Source: CAD feature listing. Evaluate the final solid. Frame: model axes, mm. Give positions to 0.01 mm unless a question says otherwise; leave off trailing zeros. Order: outer loops, then holes, each group sorted by start corner. A loop starts at its lowest first (then second) coordinate and runs counter-clockwise, first axis right, second up.
1) Section A-A, the plane x = 0. Return loops of the section in (y, z).
2) Section B-B, the plane z = 5.5. Return loops of the section in (x, y), plus the area to 3 significant figures.
3) Draft query along X for faces 1 (the face through (-2, 3.5, -2)), 2 (the face through (1.07, 1.73, -8.13)), 3 (the face through (-3, 2, 3)). Return one class per face: released by +X, released by -X, zero draft, split by the parting line, or undercut.
4) Material intervals for line 1 (Z direction, x = 0, y = 1.95); line 2 (X direction, y = 1.4, z = 6); line 3 (X direction, y = 2.25, z = 1.5), sorted ascending.
5) First-contact query: P1, Ø2, axis at x = 3.5, y = 1, coming from the +Z side; P2, Ø1, axis at x = -3.5, y = 2.5, coming from the +Z side. Flat tips, straight axial feed; report the tip coordinate or a pass-through.
6) Section D-D, the plane y = 2.35. Give the number of separate pieces and of enclosed holes in the cut face, plus the area to 3 significant figures.
7) Section C-C, the plane z = -3.75. Return loops of the section in (x, y).
Autodesk Inventor part; units mm, degrees
ref_plane "YZ Plane" through (0, 0, 0) normal (1, 0, 0) x (0, 1, 0)
ref_plane "XZ Plane" through (0, 0, 0) normal (0, 1, 0) x (-1, 0, 0)
ref_plane "XY Plane" through (0, 0, 0) normal (0, 0, 1) x (1, 0, 0)
sketch "스케치1" plane through (0, 0, 0) normal (0, 1, 0) x (-1, 0, 0)
  circle A0 centre (0, 0) radius 2.05
  line L0 (0, 0) -> (0, -15.8678) construction
  circle A1 centre (0, -5.5) radius 2.05
  line L1 (0, 0) -> (12.4059, -9.8934) construction
  circle A2 centre (4.3001, -3.4292) radius 2.05
  line L2 (0, 0) -> (15.4699, 3.5309) construction
  circle A3 centre (5.3621, 1.2239) radius 2.05
  line L3 (0, 0) -> (6.8848, 14.2964) construction
  circle A4 centre (2.3864, 4.9553) radius 2.05
  line L4 (0, 0) -> (-6.8848, 14.2964) construction
  circle A5 centre (-2.3864, 4.9553) radius 2.05
  line L5 (0, 0) -> (-15.4699, 3.5309) construction
  circle A6 centre (-5.3621, 1.2239) radius 2.05
  line L6 (0, 0) -> (-12.4059, -9.8934) construction
  circle A7 centre (-4.3001, -3.4292) radius 2.05
  circle A8 centre (0, 0) radius 8.2
  dimension "d0" = 4.1
  dimension "d2" = 4.1
  dimension "d3" = 5.5
  dimension "d6" = 360
  dimension "d8" = 16.4
extrude "돌출1" add sketch "스케치1" along normal blind 3.5
properties part number "braided_terminal_end_4.1mm_8ea"
From the geometry:
1. outline: (0, -8.2) - (3.5, -8.2) - (3.5, -7.55) - (0, -7.55) - close; (0, -3.45) - (3.5, -3.45) - (3.5, -2.05) - (0, -2.05) - close; (0, 2.05) - (3.5, 2.05) - (3.5, 8.2) - (0, 8.2) - close
2. outline: (-6.08, 0) - (-4.36, 0) - (-4.36, 3.5) - (-6.08, 3.5) - close; (-0.41, 0) - (0.41, 0) - (0.41, 3.5) - (-0.41, 3.5) - close; (4.36, 0) - (6.08, 0) - (6.08, 3.5) - (4.36, 3.5) - close
2. area: 14.9 mm2
3. face 1: zero draft
3. face 2: split by the parting line
3. face 3: undercut
4. line 1: z = -8.2 to -7.55, -3.45 to -2.05, 2.05 to 8.2
4. line 2: x = -5.59 to -4.15, -0.62 to 0.62, 4.15 to 5.59
4. line 3: x = -8.06 to -7.39, -3.33 to -1.4, 1.4 to 3.33, 7.39 to 8.06
5. P1: stops at z = 7.81
5. P2: stops at z = 7.63
6. separate pieces: 1
6. enclosed holes: 8
6. area: 106 mm2
7. outline: (-7.29, 0) - (-6.32, 0) - (-6.32, 3.5) - (-7.29, 3.5) - close; (-2.28, 0) - (-1.07, 0) - (-1.07, 3.5) - (-2.28, 3.5) - close; (1.07, 0) - (2.28, 0) - (2.28, 3.5) - (1.07, 3.5) - close; (6.32, 0) - (7.29, 0) - (7.29, 3.5) - (6.32, 3.5) - close
